Geometry check sheet. Reference: the model listing, model coordinates, mm. Round coordinates to 2 decimals unless told otherwise and drop trailing zeros. Write each loop counter-clockwise with the first axis right and the second up, starting at its lowest first coordinate (ties: lowest second). Pieces come first, ordered by that corner, then holes.
Item 1: Cross-section at A-A (y = 25). Enter the section's corners in (x, z).
Item 2: Cross-section at B-B (x = 30.5). Enter the section's corners in (y, z), then the cut area to 3 significant figures.
Item 3: Scan lines: probe 1 along X at (y, z) = (30, 0.9); probe 2 along Y at (x, z) = (25, 1); probe 3 along Y at (x, z) = (45.35, 1.3). Record each from-to range of solid material in increasing order.
Item 4: Draft check along X on faces 1 (the face through (26.18, 1.08, 0.99)), 2 (the face through (-54.57, -54, 1.01)), 3 (the face through (54.5, -54.07, 1.01)), 4 (the face through (-23.82, 1.08, 0.99)). Enter one of: pulls with the +X half, pulls with the -X half, needs draft (parallel to the pull), parting line crosses it, or undercut.
Item 5: Depth check by flat-ended pin: P1, Ø1, axis at x = -52.5, z = 1.5, coming from the +Y side; P2, Ø0.6, axis at x = -53.5, z = 1, coming from the -Y side; P3, Ø1, axis at y = -52, z = 1, coming from the +X side. Enter the tip coordinate at first touch or a pass-through.
Item 6: Cross-section at D-D (y = -22). Enter the section's corners in (x, z), then the cut area to 3 significant figures.
Item 7: Cross-section at C-C (x = -25). Enter the section's corners in (y, z), then the cut area to 3 significant figures.
from build123d import *

# Parameters (mm, degrees)
SKETCH_1_W          = 112
SKETCH_1_H          = 111
EXTRUDE_1_DEPTH     = 2
SKETCH_2_R          = 1.6
CUT_EXTRUDE_1_DEPTH = 3
SKETCH_3_W          = 2.1
SKETCH_3_H          = 23
SKETCH_3_W_2        = 23
SKETCH_3_H_2        = 2.1
CUT_EXTRUDE_2_DEPTH = 3
SKETCH_4_R          = 1.6
CUT_EXTRUDE_3_DEPTH = 3
FILLET_1_R          = 5


with BuildPart() as part:
    # 草图1 → 凸台-拉伸1 (new body)
    with BuildSketch(Plane.XY):
        Rectangle(SKETCH_1_W, SKETCH_1_H)
    extrude(amount=EXTRUDE_1_DEPTH)

    # 草图2 → 切除-拉伸1 (cut, through all)
    with BuildSketch(Plane(origin=(0, 0, 0), x_dir=(-1, 0, 0), z_dir=(0, 0, -1))):
        with Locations((-45.35, -47.55)):
            Circle(SKETCH_2_R)
        with Locations((45.35, -47.55)):
            Circle(SKETCH_2_R)
        with Locations((45.35, 47.55)):
            Circle(SKETCH_2_R)
        with Locations((-45.35, 47.55)):
            Circle(SKETCH_2_R)
    extrude(amount=-CUT_EXTRUDE_1_DEPTH, mode=Mode.SUBTRACT)

    # 草图3 → 切除-拉伸2 (cut, through all)
    with BuildSketch(Plane(origin=(0, 0, 0), x_dir=(-1, 0, 0), z_dir=(0, 0, -1))):
        with Locations((-52.9, 24)):
            Rectangle(SKETCH_3_W, SKETCH_3_H)
        with Locations((-52.9, -24)):
            Rectangle(SKETCH_3_W, SKETCH_3_H)
        with Locations((52.9, -24)):
            Rectangle(SKETCH_3_W, SKETCH_3_H)
        with Locations((52.9, 24)):
            Rectangle(SKETCH_3_W, SKETCH_3_H)
        with Locations((-24.5, -52.05)):
            Rectangle(SKETCH_3_W_2, SKETCH_3_H_2)
        with Locations((24.5, -52.05)):
            Rectangle(SKETCH_3_W_2, SKETCH_3_H_2)
        with Locations((24.5, 52.05)):
            Rectangle(SKETCH_3_W_2, SKETCH_3_H_2)
        with Locations((-24.5, 52.05)):
            Rectangle(SKETCH_3_W_2, SKETCH_3_H_2)
    extrude(amount=-CUT_EXTRUDE_2_DEPTH, mode=Mode.SUBTRACT)

    # 草图4 → 切除-拉伸3 (cut, through all)
    with BuildSketch(Plane(origin=(0, 0, 0), x_dir=(-1, 0, 0), z_dir=(0, 0, -1))):
        with Locations((-25, -25)):
            Circle(SKETCH_4_R)
        with Locations((25, -25)):
            Circle(SKETCH_4_R)
        with Locations((25, 0)):
            Circle(SKETCH_4_R)
        with Locations((25, 25)):
            Circle(SKETCH_4_R)
        with Locations((-25, 0)):
            Circle(SKETCH_4_R)
        with Locations((-25, 25)):
            Circle(SKETCH_4_R)
    extrude(amount=-CUT_EXTRUDE_3_DEPTH, mode=Mode.SUBTRACT)

    # 圆角1
    fillet_1_edges = [part.edges().sort_by_distance(p)[0] for p in [
        (56, -55.5, 1),
        (-56, -55.5, 1),
        (-56, 55.5, 1),
        (56, 55.5, 1),
    ]]
    fillet(fillet_1_edges, radius=FILLET_1_R)


solid = part.part
Resolved:
1. outline: (-56, 0) - (-53.95, 0) - (-53.95, 2) - (-56, 2) - close; (-51.85, 0) - (-26.6, 0) - (-26.6, 2) - (-51.85, 2) - close; (-23.4, 0) - (23.4, 0) - (23.4, 2) - (-23.4, 2) - close; (26.6, 0) - (51.85, 0) - (51.85, 2) - (26.6, 2) - close; (53.95, 0) - (56, 0) - (56, 2) - (53.95, 2) - close
2. outline: (-55.5, 0) - (-53.1, 0) - (-53.1, 2) - (-55.5, 2) - close; (-51, 0) - (51, 0) - (51, 2) - (-51, 2) - close; (53.1, 0) - (55.5, 0) - (55.5, 2) - (53.1, 2) - close
2. area: 214 mm2
3. probe 1: x = -56 to -53.95, -51.85 to 51.85, 53.95 to 56
3. probe 2: y = -55.5 to -53.1, -51 to -26.6, -23.4 to -1.6, 1.6 to 23.4, 26.6 to 51, 53.1 to 55.5
3. probe 3: y = -55.5 to -49.15, -45.95 to 45.95, 49.15 to 55.5
4. face 1: undercut
4. face 2: pulls with the -X half
4. face 3: pulls with the +X half
4. face 4: undercut
5. P1: stops at y = 55.4
5. P2: stops at y = -54.99
5. P3: stops at x = 55.9
6. outline: (-56, 0) - (-53.95, 0) - (-53.95, 2) - (-56, 2) - close; (-51.85, 0) - (51.85, 0) - (51.85, 2) - (-51.85, 2) - close; (53.95, 0) - (56, 0) - (56, 2) - (53.95, 2) - close
6. area: 216 mm2
7. outline: (-55.5, 0) - (-53.1, 0) - (-53.1, 2) - (-55.5, 2) - close; (-51, 0) - (-26.6, 0) - (-26.6, 2) - (-51, 2) - close; (-23.4, 0) - (-1.6, 0) - (-1.6, 2) - (-23.4, 2) - close; (1.6, 0) - (23.4, 0) - (23.4, 2) - (1.6, 2) - close; (26.6, 0) - (51, 0) - (51, 2) - (26.6, 2) - close; (53.1, 0) - (55.5, 0) - (55.5, 2) - (53.1, 2) - close
7. area: 194 mm2
